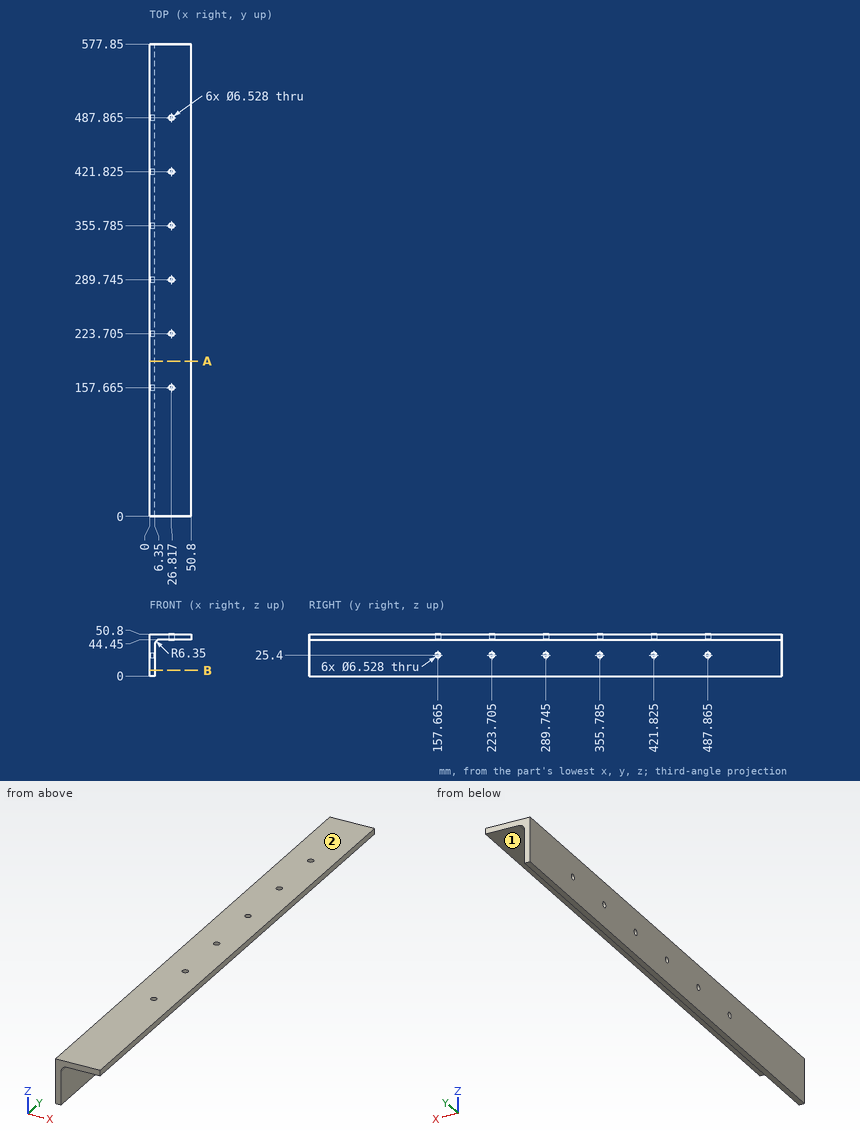
The figure shows three views and two pictorial views of one solid part (mm, origin at its lowest corner). Answer the questions. A direction names the side the tool comes from. Round coordinates to 2 decimals unless told otherwise and drop trailing zeros. Order: outer loops, then holes, each group sorted by start corner. A loop starts at its lowest first (then second) coordinate and runs counter-clockwise, first axis right, second up. Notation, with made-up numbers: M 88,-29 L 117,-29 A6 ccw 117,-22 Z; hole C 16.5,71.5 d6. An arc over 180 degrees is marked long. Answer in a Markdown table with one row per item. Add a question column.
1) Consider line 1 along Z through (x, y) = (28, 239); line 2 along X through (y, z) = (467.5, 27). Determine where each line is inside the solid, lowest interval first. Write a range as from..to.
2) The part is cut by section A-A on y = 190. Determine the outline of the cut face in (x, z).
3) Flat-ended cylindrical pins translate along their axes: pin 1 Ø4 at (x, y) = (7.5, 270) entering from -Z; pin 2 Ø19 at (y, z) = (163.5, 21.5) entering from +X; pin 3 Ø6 at (y, z) = (124.5, 31.5) entering from +X. Find the tip coordinate at first contact, or state that the pin passes through.
4) The part is cut by section B-B on z = 7. Determine the outline of the cut face in (x, y).
5) Which of the six approach directions +Z, -Z, +X, -X, +Y, -Y give full straight-line access (tool end or side, diameter ignored) to the marked faces 1 and 2?
Findings below:
| question | item | result |
|---|---|---|
| 1 | line 1 | z = 44.45..50.8 |
| 1 | line 2 | x = 0..6.35 |
| 2 | outline | M 0,0 L 6.35,0 L 6.35,38.1 A6.35 cw 12.7,44.45 L 50.8,44.45 L 50.8,50.8 L 0,50.8 Z |
| 3 | pin 1 | stops at z = 0 |
| 3 | pin 2 | stops at x = 6.35 |
| 3 | pin 3 | stops at x = 6.35 |
| 4 | outline | M 0,0 L 6.35,0 L 6.35,577.85 L 0,577.85 Z |
| 5 | face 1 | -Z, +X, +Y, -Y |
| 5 | face 2 | +Z, +X, -X, +Y, -Y |
